Source: CAD feature listing. Evaluate the final solid. Frame: model axes, mm. Face numbers are marked on the shaded views. A direction names the side the tool comes from. Round coordinates to 2 decimals unless told otherwise and drop trailing zeros. Loops run counter-clockwise (first coordinate to the right, second up) from the corner with the lowest first, then second, coordinate; pieces in that order, holes last. Notation, with made-up numbers: (31.25, -35) -> (61.25, -35) arc R34 cw to (61.25, 2) -> close; hole circle Ø8 at (15.25, 25.25). An arc over 180 degrees is marked (long way). Put each result on its own line as item: value. Start each with the question number.
1. Cut plane D-D (x = -7.75). Return the cut outline in (y, z), then the cut area to 4 significant figures.
2. Set-up query: the marked faces 1 and 2. Return all of +Z, -Z, +X, -X, +Y, -Y with unobstructed straight access to the full face (end or side cutting, diameter ignored); none if empty.
3. Contact query for a flat-ended pin moving along its axis: pin 1 (4 mm diameter, centred on x = -8.5, y = 3, fed in from -Z). Output: stop coordinate, or through.
4. Draft query along Y for the marked faces 3, 4, 5 and 6. Return one class per face: pulls with the +Y half, pulls with the -Y half, needs draft (parallel to the pull), parting line crosses it, or undercut.
5. Material intervals for L1, parallel to Y at x = 1.5, z = -1.5; L2, parallel to X at y = -7, z = 8; L3, parallel to X at y = -8, z = -1.5, sorted ascending.
6. Cut plane C-C (x = 1.75). Return the cut outline in (y, z).
7. Cut plane A-A (y = -8.5). Return the cut outline in (x, z).
8. Cut plane B-B (z = -2.25). Return the cut outline in (x, y), then the cut area to 3 significant figures.
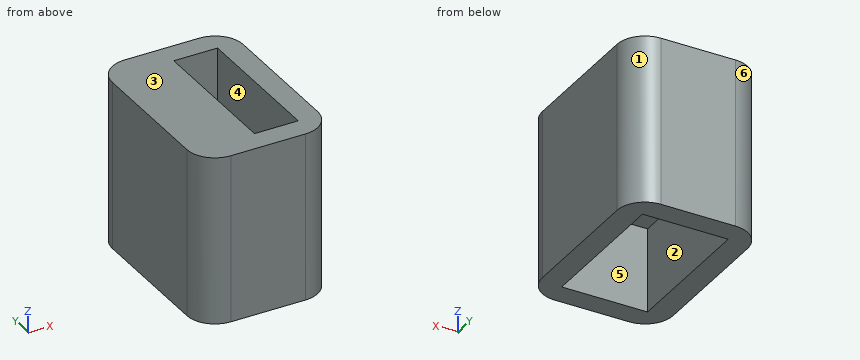
```python
from build123d import *

# Parameters (mm, degrees)
F0_W     = 15.8
F0_H     = 33.3
F0_W_2   = 7.8
F0_H_2   = 25.3
F1_DEPTH = 15
F3_DEPTH = 15
F4_DEPTH = 15
F2_W     = 3.5
F2_H     = 25.3
F5_DEPTH = 15
F6_R     = 5


with BuildPart() as f1:
    # F0 (on Top) → F1 (new body)
    with BuildSketch(Plane.XY):
        Rectangle(F0_W, F0_H)
        Rectangle(F0_W_2, F0_H_2, mode=Mode.SUBTRACT)
    extrude(amount=F1_DEPTH)

    # F2 (on Top) → F3 (join)
    with BuildSketch(Plane.XY):
        Polygon((3.9, 12.65), (3.9, -12.65), (-7.9, -12.65), (-7.9, -16.65), (5.9, -16.65), (5.9, 16.65), (-7.9, 16.65), (-7.9, 12.65), align=None)
        Polygon((-7.9, -16.65), (-7.9, -12.65), (-11.4, -12.65), (-11.4, 12.65), (-7.9, 12.65), (-7.9, 16.65), (-15.4, 16.65), (-15.4, -16.65), align=None)
    extrude(amount=-F3_DEPTH)

    # F4 (add, through all): a face of the model
    f4_faces = [f1.faces().sort_by_distance(p)[0] for p in [
        (6.9, 0, 0),
    ]]
    extrude(f4_faces, amount=F4_DEPTH)

    # F2 (on Top) → F5 (join, through all)
    with BuildSketch(Plane.XY):
        Polygon((-7.9, -16.65), (-7.9, -12.65), (-11.4, -12.65), (-11.4, 12.65), (-7.9, 12.65), (-7.9, 16.65), (-15.4, 16.65), (-15.4, -16.65), align=None)
        with Locations((-9.65, 0)):
            Rectangle(F2_W, F2_H)
    extrude(amount=F5_DEPTH)

    # F6
    f6_edges = [f1.edges().sort_by_distance(p)[0] for p in [
        (-15.4, -16.65, 0),
        (-15.4, 16.65, 0),
        (7.9, 16.65, 0),
        (7.9, -16.65, 0),
    ]]
    fillet(f6_edges, radius=F6_R)


solid = f1.part
```
Solution:
1. outline: (-16.65, -15) -> (-12.65, -15) -> (-12.65, 0) -> (12.65, 0) -> (12.65, -15) -> (16.65, -15) -> (16.65, 15) -> (-16.65, 15) -> close
1. area: 619.5 mm^2
2. face 1: +Z, -Z, +X, +Y
2. face 2: -Z
3. pin 1: stops at z = 0
4. face 3: needs draft
4. face 4: undercut
4. face 5: undercut
4. face 6: pulls with the +Y half
5. L1: y = -16.65 to -12.65, 12.65 to 16.65
5. L2: x = -15.4 to -3.9, 3.9 to 7.9
5. L3: x = -15.4 to -11.4, 3.9 to 7.9
6. outline: (-16.65, -15) -> (-12.65, -15) -> (-12.65, 15) -> (-16.65, 15) -> close; (12.65, -15) -> (16.65, -15) -> (16.65, 15) -> (12.65, 15) -> close
7. outline: (-15.4, -15) -> (-11.4, -15) -> (-11.4, 0) -> (-3.9, 0) -> (-3.9, 15) -> (-15.4, 15) -> close; (3.9, -15) -> (7.9, -15) -> (7.9, 15) -> (3.9, 15) -> close
8. outline: (-15.4, -11.65) arc R5 ccw to (-10.4, -16.65) -> (2.9, -16.65) arc R5 ccw to (7.9, -11.65) -> (7.9, 11.65) arc R5 ccw to (2.9, 16.65) -> (-10.4, 16.65) arc R5 ccw to (-15.4, 11.65) -> close; hole (-11.4, -12.65) -> (3.9, -12.65) -> (3.9, 12.65) -> (-11.4, 12.65) -> close
8. area: 367 mm^2
